Model file for the job. Use its own axes, mm. Face numbers are marked on the shaded views. A direction names the side the tool comes from. Coordinates: 2 decimals unless noted, no trailing zeros. Write each loop counter-clockwise with the first axis right and the second up, starting at its lowest first coordinate (ties: lowest second). Pieces come first, ordered by that corner, then holes. Notation, with made-up numbers: M 24.5,-34.75 L 58.5,-34.75 A28 ccw 58.5,0.25 Z; hole C -25,20 d5. An arc over 180 degrees is marked long. One line per question, with ' | ' between items. Start each with the question number.
(1) Flat gauge pins, fed straight in: pin 1 Ø4 at (x, y) = (-1.5, -16.025) entering from -Z; pin 2 Ø5.5 at (y, z) = (-8, -16) entering from -X (3 decimals); pin 3 Ø4 at (y, z) = (16.5, -27) entering from -X (3 decimals). Where does each tip first touch, or does it go through?
(2) Cut at D-D (x = 1.5). Write the cut outline in (y, z), plus the area to 3 significant figures.
(3) Cut at C-C (z = -33). Write the cut outline in (x, y) (3 decimals), plus the area to 3 significant figures.
(4) Cut at B-B (y = 17.5). Write the cut outline in (x, z) (3 decimals), plus the area to 3 significant figures.
(5) Wall check: probe 1 along Y at (x, z) = (13.7, -33); probe 2 along Y at (x, z) = (-1.5, -22.95) (3 decimals); probe 3 along Z at (x, y) = (-4, -13). Give the ranges that are in metal, low to high.
(6) Two-plate mould, pull along Z, no slides. Class the marked faces 4, 5, 6 and 7: +Z half, -Z half, draft (parallel to the pull), parting line (faces both ways), or undercut.
(7) Tool access for the marked faces 1, 2 and 3: list every direction of +Z, -Z, +X, -X, +Y, -Y with a clear straight run to the whole face (end or side of a thin tool).
(8) Cut at A-A (x = -1.5). Write the cut outline in (y, z) (3 decimals).
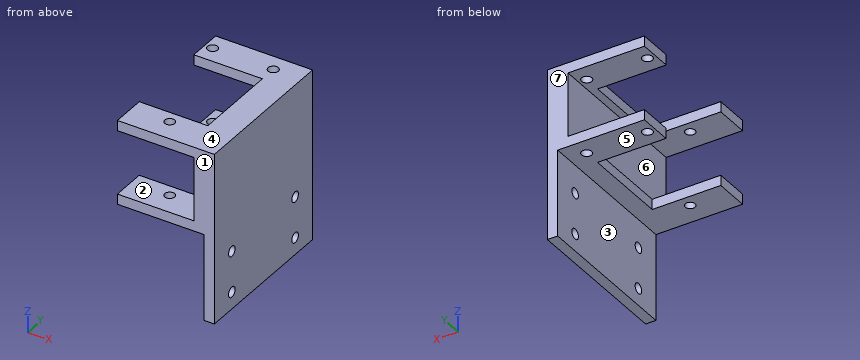
from build123d import *

# Parameters (mm, degrees)
SKETCH2_W           = 5.3
SKETCH2_H           = 25
SKETCH2_R           = 1.5
SKETCH2_R_2         = 1.445
BOSS_EXTRUDE1_DEPTH = 3
SKETCH3_W           = 50
SKETCH3_H           = 45
BOSS_EXTRUDE2_DEPTH = 3
SKETCH7_W           = 38.35
SKETCH7_H           = 3
BOSS_EXTRUDE3_DEPTH = 45
CUT_EXTRUDE1_DEPTH  = 5
SKETCH14_R          = 1.5
SKETCH14_R_2        = 1.45
CUT_EXTRUDE5_DEPTH  = 5
SKETCH15_R          = 1.5
CUT_EXTRUDE6_DEPTH  = 5
SKETCH12_W          = 18.7
SKETCH12_H          = 45
BOSS_EXTRUDE4_DEPTH = 3


with BuildPart() as part:
    # Sketch2 → Boss-Extrude1 (new body)
    # profile 1 of 3: a face of its own
    with BuildSketch(Plane.XY):
        with Locations((10.025, 0)):
            Rectangle(SKETCH2_W, SKETCH2_H)
    # profile 2 of 3: a face of its own
    with BuildSketch(Plane.XY):
        Polygon((7.375, 12.5), (12.675, 12.5), (12.675, 22.5), (-12.675, 22.5), (-12.675, 12.5), align=None)
        with Locations((-10.375, 17.5)):
            Circle(SKETCH2_R, mode=Mode.SUBTRACT)
        with Locations((7.375, 17.5)):
            Circle(SKETCH2_R, mode=Mode.SUBTRACT)
    # profile 3 of 3: a face of its own
    with BuildSketch(Plane.XY):
        Polygon((-12.675, -22.5), (12.675, -22.5), (12.675, -12.5), (7.375, -12.5), (-12.675, -12.5), align=None)
        with Locations((-1.5, -16.025)):
            Circle(SKETCH2_R_2, mode=Mode.SUBTRACT)
    extrude(amount=-BOSS_EXTRUDE1_DEPTH)

    # Sketch3 → Boss-Extrude2 (add)
    with BuildSketch(Plane(origin=(12.675, 0, 0), x_dir=(0, 0, -1), z_dir=(1, 0, 0))):
        with Locations((25, 0)):
            Rectangle(SKETCH3_W, SKETCH3_H)
    extrude(amount=BOSS_EXTRUDE2_DEPTH)

    # Sketch7 → Boss-Extrude3 (add)
    with BuildSketch(Plane(origin=(0, 22.5, 0), x_dir=(1, 0, 0), z_dir=(0, 1, 0))):
        with Locations((-3.5, 23.2)):
            Rectangle(SKETCH7_W, SKETCH7_H)
    extrude(amount=-BOSS_EXTRUDE3_DEPTH)

    # Sketch8 → Cut-Extrude1 (cut)
    with BuildSketch(Plane.XY.offset(-21.7)):
        Polygon((-12.675, 12.572802409), (-12.675, 22.5), (-22.675, 22.5), (-22.675, -22.5), (-12.675, -22.5), (-12.675, -12.5), (7.375, -12.5), (7.375, 12.572802409), align=None)
    extrude(amount=-CUT_EXTRUDE1_DEPTH, mode=Mode.SUBTRACT)

    # Sketch14 → Cut-Extrude5 (cut)
    with BuildSketch(Plane.XY.offset(-21.7)):
        with Locations((-10.375, 17.5)):
            Circle(SKETCH14_R)
        with Locations((7.375, 17.5)):
            Circle(SKETCH14_R)
        with Locations((-1.5, -16.025)):
            Circle(SKETCH14_R_2)
    extrude(amount=-CUT_EXTRUDE5_DEPTH, mode=Mode.SUBTRACT)

    # Sketch15 → Cut-Extrude6 (cut)
    with BuildSketch(Plane.ZY.offset(-12.675)):
        with Locations((-33, 14.5)):
            Circle(SKETCH15_R)
        with Locations((-33, -14.5)):
            Circle(SKETCH15_R)
        with Locations((-45, 14.5)):
            Circle(SKETCH15_R)
        with Locations((-45, -14.5)):
            Circle(SKETCH15_R)
    extrude(amount=-CUT_EXTRUDE6_DEPTH, mode=Mode.SUBTRACT)

    # Sketch12 → Boss-Extrude4 (add)
    with BuildSketch(Plane.ZY.offset(-12.675)):
        with Locations((-12.35, 0)):
            Rectangle(SKETCH12_W, SKETCH12_H)
    extrude(amount=BOSS_EXTRUDE4_DEPTH)


solid = part.part
Filled in:
1) pin 1: z = -24.7 | pin 2: x = 9.675 | pin 3: x = 12.675
2) outline: M -22.5,-24.7 L -12.5,-24.7 L -12.5,-21.7 L -22.5,-21.7 Z; M -22.5,-3 L -12.5,-3 L -12.5,0 L -22.5,0 Z; M 12.5,-3 L 22.5,-3 L 22.5,0 L 12.5,0 Z; M 12.57,-24.7 L 22.5,-24.7 L 22.5,-21.7 L 12.57,-21.7 Z | area: 120 mm²
3) outline: M 12.675,-22.5 L 15.675,-22.5 L 15.675,-16 L 12.675,-16 Z; M 12.675,-13 L 15.675,-13 L 15.675,13 L 12.675,13 Z; M 12.675,16 L 15.675,16 L 15.675,22.5 L 12.675,22.5 Z | area: 117 mm²
4) outline: M -12.675,-24.7 L -11.875,-24.7 L -11.875,-21.7 L -12.675,-21.7 Z; M -12.675,-3 L -11.875,-3 L -11.875,0 L -12.675,0 Z; M -8.875,-24.7 L 5.875,-24.7 L 5.875,-21.7 L -8.875,-21.7 Z; M -8.875,-3 L 5.875,-3 L 5.875,0 L -8.875,0 Z; M 8.875,-24.7 L 12.675,-24.7 L 12.675,-50 L 15.675,-50 L 15.675,0 L 8.875,0 L 8.875,-3 L 9.675,-3 L 9.675,-21.7 L 8.875,-21.7 Z | area: 322 mm²
5) probe 1: -22.5 to -16, -13 to 13, 16 to 22.5 | probe 2: -22.5 to -17.475, -14.575 to -12.5, 12.573 to 22.5 | probe 3: -24.7 to -21.7, -3 to 0
6) face 4: +Z half | face 5: -Z half | face 6: undercut | face 7: draft
7) face 1: +Z, -Z, +X, -X, -Y | face 2: -X, +Y, -Y | face 3: -Z, -X, +Y, -Y
8) outline: M -22.5,-24.7 L -17.475,-24.7 L -17.475,-21.7 L -22.5,-21.7 Z; M -22.5,-3 L -17.47,-3 L -17.47,0 L -22.5,0 Z; M -14.58,-3 L -12.5,-3 L -12.5,0 L -14.58,0 Z; M -14.575,-24.7 L -12.5,-24.7 L -12.5,-21.7 L -14.575,-21.7 Z; M 12.5,-3 L 22.5,-3 L 22.5,0 L 12.5,0 Z; M 12.573,-24.7 L 22.5,-24.7 L 22.5,-21.7 L 12.573,-21.7 Z
